```python
from build123d import *

# Parameters (mm, degrees)
F1_DEPTH = 12
F2_R     = 2.5527
F3_DEPTH = 25.4


with BuildPart() as f1:
    # F0 (on Right) → F1 (new body)
    with BuildSketch(Plane.YZ):
        Polygon((-63.814045, 83.583468), (-89.214045, 83.583468), (-89.214045, -68.816532), (63.185955, -68.816532), (63.185955, -43.416532), align=None)
    extrude(amount=F1_DEPTH)

    # F2 (on face) → F3 (cut)
    with BuildSketch(Plane.YZ.offset(12)):
        with Locations((-76.514045, -56.116532)):
            Circle(F2_R)
        with Locations((-76.514045, -30.716532)):
            Circle(F2_R)
        with Locations((-76.514045, -5.316532)):
            Circle(F2_R)
        with Locations((-76.514045, 20.083468)):
            Circle(F2_R)
        with Locations((-76.514045, 45.483468)):
            Circle(F2_R)
        with Locations((-76.514045, 70.883468)):
            Circle(F2_R)
        with Locations((-51.114045, -56.116532)):
            Circle(F2_R)
        with Locations((-25.714045, -56.116532)):
            Circle(F2_R)
        with Locations((-0.314045, -56.116532)):
            Circle(F2_R)
        with Locations((25.085955, -56.116532)):
            Circle(F2_R)
        with Locations((50.485955, -56.116532)):
            Circle(F2_R)
    extrude(amount=-F3_DEPTH, mode=Mode.SUBTRACT)


solid = f1.part
```
CAD build for the part. Positions are in the model's coordinates, mm. Round coordinates to 2 decimals unless told otherwise and drop trailing zeros. Order: outer loops, then holes, each group sorted by start corner. A loop starts at its lowest first (then second) coordinate and runs counter-clockwise, first axis right, second up.
Item 1: Probe line 1 along Z through (x, y) = (10.5, -30); line 2 along Z through (x, y) = (9.5, 48.5); line 3 along Y through (x, z) = (4.75, 70). List the from-to ranges inside material, lowest first.
Item 2: Saw through at B-B on x = 5. State how many separate pieces and enclosed holes the cut face has, then the cut area to 3 significant figures.
Item 3: Saw through at D-D on y = -59.5. Write the cut outline in (x, z), then the cut area to 3 significant figures.
Item 4: Pin check, flat tips, straight feed: pin 1 (6 mm diameter, centred on x = 2, z = 41.5, fed in from +Y); pin 2 (3 mm diameter, centred on y = -51.11, z = -56.12, fed in from -X); pin 3 (4 mm diameter, centred on x = 6, y = 12.5, fed in from +Z); pin 4 (2 mm diameter, centred on x = 10.5, z = 67, fed in from +Y). Stop position of each tip, or through.
Item 5: Saw through at C-C on z = 27.5. Write the cut outline in (x, y).
Item 6: Mould opens along Y. For faces 1 (the face through (6, 63.186, -56)), 2 (the face through (6, -14, -68.817)), 3 (the face through (6.084, 26.264, -58.381)), 4 (the face through (6, -89.214, 8)) say: pulls with the +Y half, pulls with the -Y half, needs draft (parallel to the pull), parting line crosses it, or undercut.
Item 7: Saw through at A-A on y = -26. Write the cut outline in (x, z).
Reported:
1. line 1: z = -68.82 to 49.77
1. line 2: z = -68.82 to -57.72, -54.51 to -28.73
1. line 3: y = -89.21 to -78.91, -74.12 to -50.23
2. separate pieces: 1
2. enclosed holes: 11
2. area: 14,900 mm2
3. outline: (0, -68.82) - (12, -68.82) - (12, 79.27) - (0, 79.27) - close
3. area: 1,780 mm2
4. pin 1: stops at y = -18.73
4. pin 2: passes through
4. pin 3: stops at z = 9.27
4. pin 4: stops at y = -46.23
5. outline: (0, -89.21) - (12, -89.21) - (12, -7.73) - (0, -7.73) - close
6. face 1: pulls with the +Y half
6. face 2: needs draft
6. face 3: undercut
6. face 4: pulls with the -Y half
7. outline: (0, -68.82) - (12, -68.82) - (12, -58.65) - (0, -58.65) - close; (0, -53.58) - (12, -53.58) - (12, 45.77) - (0, 45.77) - close
